Part model, mm, in its own coordinate system. Face numbers are marked on the shaded views. A direction names the side the tool comes from. Give positions to 0.01 mm unless a question says otherwise; leave off trailing zeros. Write each loop counter-clockwise with the first axis right and the second up, starting at its lowest first coordinate (ties: lowest second). Pieces come first, ordered by that corner, then holes.
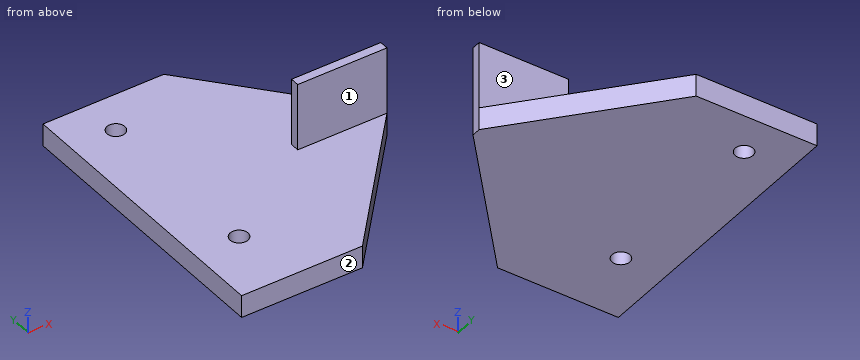
from build123d import *

# Parameters (mm, degrees)
SKETCH1_W           = 54.124737276
SKETCH1_H           = 64.519725693
SKETCH1_R           = 2
BOSS_EXTRUDE1_DEPTH = 5
SKETCH7_W           = 20
SKETCH7_H           = 2
BOSS_EXTRUDE4_DEPTH = 20
CUT_EXTRUDE4_DEPTH  = 7


with BuildPart() as part:
    # Sketch1 → Boss-Extrude1 (new body)
    with BuildSketch(Plane.XY):
        with Locations((-293.137631362, -203.073045314)):
            Rectangle(SKETCH1_W, SKETCH1_H)
        with Locations((-310.2, -180)):
            Circle(SKETCH1_R, mode=Mode.SUBTRACT)
        with Locations((-310.2, -220)):
            Circle(SKETCH1_R, mode=Mode.SUBTRACT)
    extrude(amount=BOSS_EXTRUDE1_DEPTH)

    # Sketch7 → Boss-Extrude4 (add)
    with BuildSketch(Plane(origin=(-266.075262724, 0, 0), x_dir=(0, 0, -1), z_dir=(1, 0, 0))):
        with Locations((-10, -203.073045313)):
            Rectangle(SKETCH7_W, SKETCH7_H)
    extrude(amount=-BOSS_EXTRUDE4_DEPTH)

    # Sketch8 → Cut-Extrude4 (cut)
    with BuildSketch(Plane.XY.offset(5)):
        Polygon((-266.075262724, -204.073045313), (-293.137631362, -235.33290816), (-266.075262724, -235.33290816), align=None)
        Polygon((-293.137631362, -170.813182467), (-266.075262724, -202.073045313), (-266.075262724, -170.813182467), align=None)
    extrude(amount=-CUT_EXTRUDE4_DEPTH, mode=Mode.SUBTRACT)


solid = part.part
1) Saw through at B-B (z = 1.75). Write the cut outline in (x, y).
Check result:
outline: (-320.2, -235.33) - (-293.14, -235.33) - (-266.08, -204.07) - (-266.08, -202.07) - (-293.14, -170.81) - (-320.2, -170.81) - close; hole circle Ø4 at (-310.2, -220); hole circle Ø4 at (-310.2, -180)
2) Drill centre lines: L1, parallel to Y at x = -310.2, z = 2; L2, parallel to Z at x = -299, y = -187.5; L3, parallel to X at y = -220, z = 2.35. Where is each one in solid material? Low to high.
Check result:
L1: y = -235.33 to -222, -218 to -182, -178 to -170.81
L2: z = 0 to 5
L3: x = -320.2 to -312.2, -308.2 to -279.86
3) Flat gauge pins, fed straight in: P1, Ø4.5, axis at x = -279, z = 10.5, coming from the -Y side; P2, Ø3.5, axis at x = -310.2, y = -180, coming from the +Z side (3 decimals); P3, Ø1.5, axis at x = -314.5, y = -217, coming from the -Z side; P4, Ø10, axis at y = -206, z = 12.5, coming from the -X side. Where does each tip first touch, or does it go through?
Check result:
P1: stops at y = -204.07
P2: passes through
P3: stops at z = 0
P4: stops at x = -286.08
4) Saw through at D-D (x = -276.5). Write the cut outline in (y, z), and give its area (3 significant figures).
Check result:
outline: (-216.11, 0) - (-190.03, 0) - (-190.03, 5) - (-202.07, 5) - (-202.07, 20) - (-204.07, 20) - (-204.07, 5) - (-216.11, 5) - close
area: 160 mm2
5) Saw through at A-A (x = -310.2). Write the cut outline in (y, z), and give its area (3 significant figures).
Check result:
outline: (-235.33, 0) - (-222, 0) - (-222, 5) - (-235.33, 5) - close; (-218, 0) - (-182, 0) - (-182, 5) - (-218, 5) - close; (-178, 0) - (-170.81, 0) - (-170.81, 5) - (-178, 5) - close
area: 283 mm2
6) 3-axis set-ups, long thin cutter, end or side, ignore diameter. For the marked faces 1, 2 and 3: which of +Z, -Z, +X, -X, +Y, -Y reach the whole face in a straight line?
Check result:
face 1: +Z, +X, -X, -Y
face 2: +Z, -Z, +X, -X, -Y
face 3: +Z, +X, -X, +Y
7) Saw through at C-C (y = -220). Write the cut outline in (x, z), and give its area (3 significant figures).
Check result:
outline: (-320.2, 0) - (-312.2, 0) - (-312.2, 5) - (-320.2, 5) - close; (-308.2, 0) - (-279.86, 0) - (-279.86, 5) - (-308.2, 5) - close
area: 182 mm2
